Work out the finished part from the listing and answer in its coordinate system (mm). Coordinates: 2 decimals unless noted, no trailing zeros. Order: outer loops, then holes, each group sorted by start corner. A loop starts at its lowest first (then second) coordinate and runs counter-clockwise, first axis right, second up.
1. Find the intervals of material crossed by probe 1 along Z at (x, y) = (191.5, -252.75); probe 2 along Y at (x, z) = (-83, -3.25); probe 3 along X at (y, z) = (-253.75, 4.5), in increasing order.
2. The part is cut by section B-B, the plane x = 147. Give the vertices of the cut face in (y, z).
3. The part is cut by section A-A, the plane y = -259. Give the vertices of the cut face in (x, z), then the cut area to 3 significant figures.
4. Flat-ended cylindrical pins translate along their axes: pin 1 Ø1 at (y, z) = (-257.5, -1.5) entering from -X; pin 2 Ø1 at (y, z) = (-260.5, -3) entering from -X; pin 3 Ø4 at (y, z) = (-262.5, 7) entering from -X; pin 4 Ø4 at (x, z) = (-23.5, -6) entering from +Y. Find the tip coordinate at first contact, or state that the pin passes through.
5. The part is cut by section C-C, the plane z = -4. Give the vertices of the cut face in (x, y).
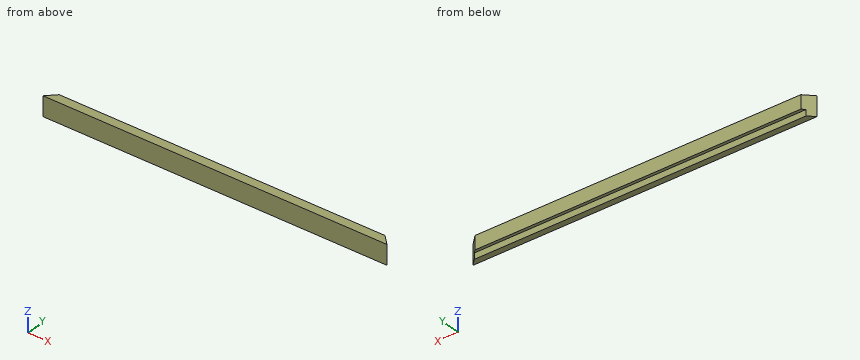
```python
from build123d import *

# Parameters (mm, degrees)
PAD003_DEPTH         = 350
POCKET002_DEPTH      = 8.001
POCKET002_DEPTH_BACK = 30.001
SKETCH008_W          = 12
SKETCH008_H          = 12
POCKET003_DEPTH      = 226.501
POCKET003_DEPTH_BACK = 226.501


with BuildPart() as part:
    # Sketch005 → Pad003 (new body, symmetric)
    with BuildSketch(Plane.YZ):
        Polygon((-252, 0), (-252, 30), (-264, 25.632357), (-264, -8), (-256, -8), (-256, 0), align=None)
    extrude(amount=PAD003_DEPTH, both=True)

    # Sketch006 → Pocket002 (cut, two sides)
    with BuildSketch(Plane.XY) as pocket002_sk:
        Polygon((-350, -264), (-350, -252), (-214.5, -252), (-226.5, -264), align=None)
        Polygon((350, -264), (350, -252), (214.5, -252), (226.5, -264), align=None)
    extrude(amount=-POCKET002_DEPTH, mode=Mode.SUBTRACT)
    extrude(pocket002_sk.sketch, amount=POCKET002_DEPTH_BACK, mode=Mode.SUBTRACT)

    # Sketch008 → Pocket003 (cut, two sides)
    with BuildSketch(Plane.YZ) as pocket003_sk:
        with Locations((-258, 24)):
            Rectangle(SKETCH008_W, SKETCH008_H)
    extrude(amount=-POCKET003_DEPTH, mode=Mode.SUBTRACT)
    extrude(pocket003_sk.sketch, amount=POCKET003_DEPTH_BACK, mode=Mode.SUBTRACT)


solid = part.part
```
Geometry says:
1. probe 1: z = 0 to 18
1. probe 2: y = -264 to -256
1. probe 3: x = -216.25 to 216.25
2. outline: (-264, -8) - (-256, -8) - (-256, 0) - (-252, 0) - (-252, 18) - (-264, 18) - close
3. outline: (-221.5, -8) - (221.5, -8) - (221.5, 18) - (-221.5, 18) - close
3. area: 11,500 mm2
4. pin 1: stops at x = -220.5
4. pin 2: stops at x = -223.5
4. pin 3: stops at x = -226.5
4. pin 4: stops at y = -256
5. outline: (-226.5, -264) - (226.5, -264) - (218.5, -256) - (-218.5, -256) - close
